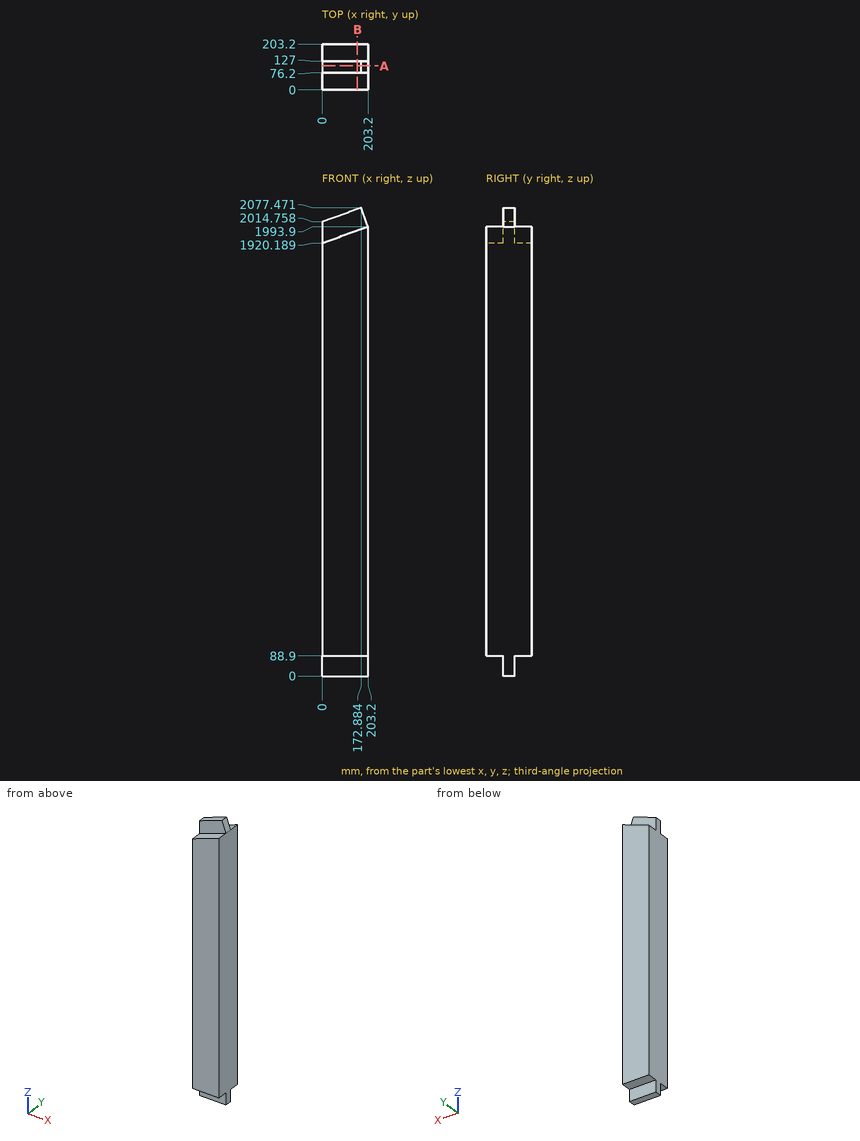
Verification items for this drawing (mm, ordinates from the low corner). Give positions to 0.01 mm unless a question says otherwise; leave off trailing zeros. Write each loop counter-clockwise with the first axis right and the second up, starting at its lowest first coordinate (ties: lowest second). Pieces come first, ordered by that corner, then holes. Notation, with made-up numbers: (78, 69.5) -> (134, 69.5) arc R24 ccw to (134, 95.5) -> close; hole circle Ø5 at (66, -11). An arc over 180 degrees is marked (long way). Write item = value, one per line.
Item 1: Sectioned sample at B-B on x = 156. Record the boundary of the cut face in (y, z), and give its area (3 significant figures).
Output:
outline = (0, 88.9) -> (76.2, 88.9) -> (76.2, 0) -> (127, 0) -> (127, 88.9) -> (203.2, 88.9) -> (203.2, 1976.78) -> (127, 1976.78) -> (127, 2071.35) -> (76.2, 2071.35) -> (76.2, 1976.78) -> (0, 1976.78) -> close
area = 393,000 mm^2
Item 2: Gauge pin test, flat end, axial feed: pin 1 (12 mm diameter, centred on x = 81, y = 136, fed in from -Z). Record the tip position at first contact, or that the pin passes through.
Output:
pin_1 = 88.9
Item 3: Sectioned sample at A-A on y = 106. Record the boundary of the cut face in (x, z) (1 decimal).
Output:
outline = (0, 0) -> (203.2, 0) -> (203.2, 1993.9) -> (172.9, 2077.5) -> (0, 2014.8) -> close
Item 4: Scan lines: probe 1 along Y at (x, z) = (39, 1939); probe 2 along Z at (x, y) = (97, 28) (1 decimal); probe 3 along Z at (x, y) = (122, 147.5) (1 decimal). Record each from-to range of solid material in increasing order. Write a range as from..to.
Output:
probe_1 = 76.2..127
probe_2 = 88.9..1955.4
probe_3 = 88.9..1964.4
